The listing builds one solid part. Answer for the finished solid, in the listing's coordinates (mm). Give positions to 0.01 mm unless a question says otherwise; leave off trailing zeros. Write each loop counter-clockwise with the first axis right and the second up, starting at its lowest first coordinate (ties: lowest second). Pieces come first, ordered by that corner, then holes. Notation, with made-up numbers: M 20.25,-34 L 77.25,-34 A18 ccw 77.25,-3 Z; hole C 55.5,42.5 d5. An arc over 180 degrees is marked long. Return JSON: item names as keys, results as strings.
Autodesk Inventor part; units mm, degrees
ref_plane "YZ Plane" through (0, 0, 0) normal (1, 0, 0) x (0, 1, 0)
ref_plane "XZ Plane" through (0, 0, 0) normal (0, 1, 0) x (-1, 0, 0)
ref_plane "XY Plane" through (0, 0, 0) normal (0, 0, 1) x (1, 0, 0)
sketch "Sketch1" plane through (0, 0, 0) normal (0, 0, 1) x (1, 0, 0)
  circle A0 centre (-83.65, 30) radius 2.1
  circle A1 centre (-23.65, 30) radius 2.1
  circle A2 centre (-23.65, 50) radius 2.1
  circle A3 centre (-83.65, 50) radius 2.1
  line L0 (-3.55, 0) -> (-3.5497, 1000)
  line L1 (16.25, 0) -> (16.2503, 1000)
  line L2 (-93.65, 20.5) -> (-93.65, 25.1685)
  line L3 (-73.65, 25.1685) -> (-73.65, 20.5)
  line L4 (-78.75, 60) -> (-68.55, 60)
  line L5 (-88.55, 20) -> (-93.15, 20)
  line L6 (-93.65, 20) -> (-93.65, 60)
  line L7 (-93.65, 60) -> (26.35, 60)
  line L8 (26.35, 60) -> (26.35, 0)
  line L9 (26.35, 0) -> (-3.55, 0)
  line L10 (-93.65, -22.5923) -> (-93.65, 20)
  line L11 (-74.15, 20) -> (-78.75, 20) construction
  line L12 (-33.65, 20.5) -> (-33.65, 25.1685)
  line L13 (-53.65, -43.196) -> (-53.65, 110.7641) construction
  line L14 (-13.65, 0) -> (-38.74, -22.5923)
  circle A4 centre (-53.65, 27.5) radius 11.1
  circle A5 centre (-43.65, 50) radius 2.1
  line L15 (-93.65, -22.5923) -> (-38.74, -22.5923)
  line L16 (-13.65, 0) -> (-3.55, 0)
  point P0 (0, 0)
  point P1 (-62.8644, -22.5923)
  point P2 (-93.65, -24.4136)
  point P3 (-3.55, 15)
  point P4 (-3.55, 50)
  point P5 (16.25, 50)
  point P6 (16.25, 15)
  dimension "d0" = 120
  dimension "d1" = 40
  dimension "d5" = 20
  dimension "d36" = 22.2
  dimension "d37" = 32.5
  dimension "d45" = 15
  dimension "d47" = 50
  dimension "d48" = 50
  dimension "d79" = 15
extrude "Extrusion2" add sketch "Sketch1" against normal blind 6 contours A0 | A1 | A2 | A3 | L16 L14 L15 L10 L6 L2 L7 L4 L0 | L0 L7 L1 L9 | L1 L7 L8 L9 | A5
ref_plane "Work Plane1" through (0, 0, 5) normal (0, 0, 1) x (1, 0, 0)
sketch "Sketch2" plane through (0, 0, 5) normal (0, 0, 1) x (1, 0, 0)
  line L0 (-66.3198, 58.2348) -> (-84.359, 14.8345) construction
  line L1 (-84.359, 14.8345) -> (-40.9587, -3.2047) construction
  line L2 (-40.9587, -3.2047) -> (-22.9195, 40.1957) construction
  line L3 (-22.9195, 40.1957) -> (-66.3198, 58.2348) construction
  line L4 (-66.3198, 58.2348) -> (-40.9587, -3.2047) construction
  line L5 (-84.359, 14.8345) -> (-22.9195, 40.1957) construction
  circle A0 centre (-22.9195, 40.1957) radius 4.6 construction
  circle A1 centre (-84.359, 14.8345) radius 4.6 construction
  point P0 (0, 0)
  point P1 (-53.6392, 27.5151)
  dimension "d41" = 47
  dimension "d42" = 47
  dimension "d43" = 9.2
  dimension "d44" = 9.2
hole "Hole2" at (-84.359, 14.8345, 5) at (-22.9195, 40.1957, 5) at (-40.9587, -3.2047, 5) direction (0, 0, -1) diameter 5.1 end through all
hole "Hole3" at (-53.65, 27.5, 0) at (-43.65, 50, 0) at (-23.65, 50, 0) at (-23.65, 30, 0) at (-83.65, 50, 0) at (-83.65, 30, 0) direction (0, 0, -1) diameter 5.1 end through all
sketch "Sketch3" plane through (0, 0, 0) normal (0, 0, 1) x (1, 0, 0)
  point P0 (0, 0)
  point P1 (-3.2825, 15.0941)
  point P2 (-3.7043, 49.839)
  point P3 (16.7382, 49.8563)
  point P4 (15.6257, 14.0035)
hole "Hole4" at (-3.2825, 15.0941, 0) at (-3.7043, 49.839, 0) at (16.7382, 49.8563, 0) at (15.6257, 14.0035, 0) direction (0, 0, -1) diameter 5.1 end through all
properties part number "Y axis motor mount new_3DPrint"
Item 1: A cutting plane is placed at B-B, the plane x = -57.5. Write down the section's boundary in (y, z), plus the area to 3 significant figures.
Geometry results:
{"outline": "M -22.59,-6 L 17.09,-6 L 17.09,0 L -22.59,0 Z; M 37.91,-6 L 60,-6 L 60,0 L 37.91,0 Z", "area": "371 mm2"}
Item 2: Find the intervals of material crossed by line 1 (X direction, y = 50, z = -4.85); line 2 (Y direction, x = -3.5, z = -2.8); line 3 (Y direction, x = -23.65, z = -3.15), in increasing order.
Geometry results:
{"line 1": "x = -93.65 to -86.2, -81.1 to -46.2, -41.1 to -26.2, -21.1 to -6.25, -1.16 to 14.19, 19.28 to 26.35", "line 2": "y = 0 to 12.55, 17.63 to 47.3, 52.38 to 60", "line 3": "y = -9 to 27.45, 32.55 to 37.75, 42.64 to 47.45, 52.55 to 60"}
Item 3: A cutting plane is placed at A-A, the plane y = 50. Write down the section's boundary in (x, z), plus the area to 3 significant figures.
Geometry results:
{"outline": "M -93.65,-6 L -86.2,-6 L -86.2,0 L -93.65,0 Z; M -81.1,-6 L -46.2,-6 L -46.2,0 L -81.1,0 Z; M -41.1,-6 L -26.2,-6 L -26.2,0 L -41.1,0 Z; M -21.1,-6 L -6.25,-6 L -6.25,0 L -21.1,0 Z; M -1.16,-6 L 14.19,-6 L 14.19,0 L -1.16,0 Z; M 19.28,-6 L 26.35,-6 L 26.35,0 L 19.28,0 Z", "area": "567 mm2"}
Item 4: A cutting plane is placed at C-C, the plane y = 35. Write down the section's boundary in (x, z).
Geometry results:
{"outline": "M -93.65,-6 L -61.83,-6 L -61.83,0 L -93.65,0 Z; M -45.47,-6 L 26.35,-6 L 26.35,0 L -45.47,0 Z"}
Item 5: Determine the mould class of faces 1 (the flat face through (6, 0, -3)), 2 (the cylindrical face through (-82.098, 52.024, -3.042)), 3 (the flat face through (26.35, 30, -3)) for opening direction Y: +Y half, -Y half, draft (parallel to the pull), parting line (faces both ways), or undercut.
Geometry results:
{"face 1": "-Y half", "face 2": "undercut", "face 3": "draft"}
Item 6: A cutting plane is placed at D-D, the plane z = -1.95. Count the separate pieces of the cut face and the enclosed holes in it, plus the area to 3 significant figures.
Geometry results:
{"separate pieces": "1", "enclosed holes": "13", "area": "8,090 mm2"}
Item 7: Given pin 1 Ø3 at (x, z) = (0, -4.5) entering from -Y; pin 2 Ø4.5 at (x, y) = (-83.65, 30) entering from +Z; pin 3 Ø2 at (y, z) = (-6, -4.5) entering from +X, each flat-ended and moving along its own axis, determine where each tip first touches the part or whether it passes through.
Geometry results:
{"pin 1": "stops at y = 0", "pin 2": "passes through", "pin 3": "stops at x = -19.2"}
